```python
from build123d import *

# Parameters (mm, degrees)
F3_R   = 7
F3_R_2 = 9


# Not quite as in the source:
# - a pattern or mirror of a feature is missing from the dataset's text; its kind, count and spacing are read off the source's solid


with BuildPart() as f1:
    # F0 (on Front) → F1 (revolve)
    with BuildSketch(Plane.XZ):
        with BuildLine():
            Line((-61, 0), (0, 0))
            Line((0, 0), (0, 10))
            add(Edge.make_bspline(
                [(-50.25, 18.6195461814), (-37.2210499958, 26.1418139735), (-10.4841707805, 16.6390100311), (-3.3322397366, 11.9742266545), (0, 10)],
                knots=[0, 0, 0, 0, 0.6387203747, 1, 1, 1, 1], degree=3))
            ThreePointArc((-50.25, 18.6195461814), (-58.1195461814, 10.75), (-61, 0))
        make_face()
    revolve(axis=Axis((-30.5, 0, 0), (-1, 0, 0)))

    # F3 (on offset) → F4 (join, up to the next surface of F1)
    with BuildSketch(Plane.XZ.offset(30)):
        with Locations((-15.8201763071, 7.2742023454)):
            Circle(F3_R)
        with Locations((-40.0313028448, 9.3763558499)):
            Circle(F3_R_2)
    f4 = extrude(until=Until.NEXT, dir=(0, 1, 0))

    # F4_copies: F4 across plane
    add(f4.mirror(Plane.ZX))


solid = f1.part
```
The listing builds one solid part. Answer for the finished solid, in the listing's coordinates (mm). A direction names the side the tool comes from. Give positions to 0.01 mm unless a question says otherwise; leave off trailing zeros. Order: outer loops, then holes, each group sorted by start corner. A loop starts at its lowest first (then second) coordinate and runs counter-clockwise, first axis right, second up.
Item 1: The part is cut by section A-A, the plane x = -57. Give the vertices of the cut face in (y, z), and give its area (3 significant figures).
From the geometry:
outline: circle Ø24.98 at (0, 0)
area: 490 mm2
Item 2: Which of the six approach directions +Z, -Z, +X, -X, +Y, -Y give full straight-line access (tool end or side, diameter ignored) to faces 5 (the face through (-40, -30, 10)), 6 (the face through (-12.06, -22.27, 13.18))?
From the geometry:
face 5: +Z, -Z, +X, -X, -Y
face 6: -Y
Item 3: Given pin 1 Ø2 at (x, z) = (-45, -6.5) entering from -Y; pin 2 Ø1.5 at (x, y) = (-33, 5.5) entering from +Z; pin 3 Ø10 at (x, y) = (-11.5, 4.5) entering from -Z, each flat-ended and moving along its own axis, determine where each tip first touches the part or whether it passes through.
From the geometry:
pin 1: stops at y = -20.29
pin 2: stops at z = 21.58
pin 3: stops at z = -17.9
Item 4: For a pull along X with two mould halves and no side action, classify faces 1 (the face through (0, 0, 0)), 2 (the face through (-12.06, 22.27, 13.18)), 3 (the face through (-16, 30, 7)), 4 (the face through (-41.2, 23, 18.3)) as pulls with the +X half, pulls with the -X half, needs draft (parallel to the pull), parting line crosses it, or undercut.
From the geometry:
face 1: pulls with the +X half
face 2: undercut
face 3: needs draft
face 4: undercut
Item 5: Find the intervals of material crossed by probe 1 along X at (y, z) = (22.5, 13); probe 2 along X at (y, z) = (10, -14); probe 3 along X at (y, z) = (3, 9.5), in increasing order.
From the geometry:
probe 1: x = -48.27 to -31.79, -19.85 to -11.79
probe 2: x = -52.39 to -13.9
probe 3: x = -58.55 to 0
